```python
from build123d import *

# Parameters (mm, degrees)
F1_DEPTH = 16
F2_T     = -2
F3_W     = 41.64
F3_H     = 10.8
F3_R     = 2.75
F4_DEPTH = 16.001
F5_R     = 1
F6_DEPTH = 5.5


with BuildPart() as f1:
    # F0 (on Top) → F1 (new body)
    with BuildSketch(Plane.XY):
        with BuildLine():
            ThreePointArc((36.115, 24.13), (33.906585, 29.461585), (28.575, 31.67))
            Line((28.575, 31.67), (-28.575, 31.67))
            ThreePointArc((-28.575, 31.67), (-33.906585, 29.461585), (-36.115, 24.13))
            Line((-36.115, 24.13), (-36.115, -24.13))
            ThreePointArc((-36.115, -24.13), (-33.906585, -29.461585), (-28.575, -31.67))
            Line((-28.575, -31.67), (28.575, -31.67))
            ThreePointArc((28.575, -31.67), (33.906585, -29.461585), (36.115, -24.13))
            Line((36.115, -24.13), (36.115, 24.13))
        make_face()
    extrude(amount=F1_DEPTH)

    # F2
    f2_openings = [f1.faces().sort_by_distance(p)[0] for p in [
        (0, 0, 16),
    ]]
    offset(amount=F2_T, openings=f2_openings)

    # F3 (on Top) → F4 (cut, through all)
    with BuildSketch(Plane.XY):
        with Locations((-0.635, -19.162)):
            Rectangle(F3_W, F3_H)
        with BuildLine():
            Line((-8.585, -0.6), (-18.085, -0.6))
            ThreePointArc((-18.085, -0.6), (-18.792107, -0.892893), (-19.085, -1.6))
            Line((-19.085, -1.6), (-19.085, -11.1))
            ThreePointArc((-19.085, -11.1), (-18.792107, -11.807107), (-18.085, -12.1))
            Line((-18.085, -12.1), (-8.585, -12.1))
            ThreePointArc((-8.585, -12.1), (-7.877893, -11.807107), (-7.585, -11.1))
            Line((-7.585, -11.1), (-7.585, -1.6))
            ThreePointArc((-7.585, -1.6), (-7.877893, -0.892893), (-8.585, -0.6))
        make_face()
        with Locations((-26.035, -6.35)):
            Circle(F3_R)
        with BuildLine():
            Line((-8.585, 20.08), (-18.085, 20.08))
            ThreePointArc((-18.085, 20.08), (-18.792107, 19.787107), (-19.085, 19.08))
            Line((-19.085, 19.08), (-19.085, 9.58))
            ThreePointArc((-19.085, 9.58), (-18.792107, 8.872893), (-18.085, 8.58))
            Line((-18.085, 8.58), (-8.585, 8.58))
            ThreePointArc((-8.585, 8.58), (-7.877893, 8.872893), (-7.585, 9.58))
            Line((-7.585, 9.58), (-7.585, 19.08))
            ThreePointArc((-7.585, 19.08), (-7.877893, 19.787107), (-8.585, 20.08))
        make_face()
        with Locations((-26.035, 14.33)):
            Circle(F3_R)
        with BuildLine():
            Line((23.165, -0.6), (13.665, -0.6))
            ThreePointArc((13.665, -0.6), (12.957893, -0.892893), (12.665, -1.6))
            Line((12.665, -1.6), (12.665, -11.1))
            ThreePointArc((12.665, -11.1), (12.957893, -11.807107), (13.665, -12.1))
            Line((13.665, -12.1), (23.165, -12.1))
            ThreePointArc((23.165, -12.1), (23.872107, -11.807107), (24.165, -11.1))
            Line((24.165, -11.1), (24.165, -1.6))
            ThreePointArc((24.165, -1.6), (23.872107, -0.892893), (23.165, -0.6))
        make_face()
        with Locations((5.715, -6.35)):
            Circle(F3_R)
        with BuildLine():
            Line((23.165, 20.08), (13.665, 20.08))
            ThreePointArc((13.665, 20.08), (12.957893, 19.787107), (12.665, 19.08))
            Line((12.665, 19.08), (12.665, 9.58))
            ThreePointArc((12.665, 9.58), (12.957893, 8.872893), (13.665, 8.58))
            Line((13.665, 8.58), (23.165, 8.58))
            ThreePointArc((23.165, 8.58), (23.872107, 8.872893), (24.165, 9.58))
            Line((24.165, 9.58), (24.165, 19.08))
            ThreePointArc((24.165, 19.08), (23.872107, 19.787107), (23.165, 20.08))
        make_face()
        with Locations((5.715, 14.33)):
            Circle(F3_R)
    extrude(amount=F4_DEPTH, mode=Mode.SUBTRACT)

    # F5 (on face) → F6 (join)
    with BuildSketch(Plane.XY.offset(2)):
        with BuildLine():
            Line((-34.115, 24.13), (-34.115, 21.59))
            Line((-34.115, 21.59), (-28.575, 21.59))
            ThreePointArc((-28.575, 21.59), (-26.778949, 22.333949), (-26.035, 24.13))
            Line((-26.035, 24.13), (-26.035, 29.67))
            Line((-26.035, 29.67), (-28.575, 29.67))
            ThreePointArc((-28.575, 29.67), (-32.492372, 28.047372), (-34.115, 24.13))
        make_face()
        with Locations((-28.575, 24.13)):
            Circle(F5_R, mode=Mode.SUBTRACT)
        with BuildLine():
            Line((28.575, 21.59), (34.115, 21.59))
            Line((34.115, 21.59), (34.115, 24.13))
            ThreePointArc((34.115, 24.13), (32.492372, 28.047372), (28.575, 29.67))
            Line((28.575, 29.67), (26.035, 29.67))
            Line((26.035, 29.67), (26.035, 24.13))
            ThreePointArc((26.035, 24.13), (26.778949, 22.333949), (28.575, 21.59))
        make_face()
        with Locations((28.575, 24.13)):
            Circle(F5_R, mode=Mode.SUBTRACT)
        with BuildLine():
            Line((26.035, -24.13), (26.035, -29.67))
            Line((26.035, -29.67), (28.575, -29.67))
            ThreePointArc((28.575, -29.67), (32.492372, -28.047372), (34.115, -24.13))
            Line((34.115, -24.13), (34.115, -21.59))
            Line((34.115, -21.59), (28.575, -21.59))
            ThreePointArc((28.575, -21.59), (26.778949, -22.333949), (26.035, -24.13))
        make_face()
        with Locations((28.575, -24.13)):
            Circle(F5_R, mode=Mode.SUBTRACT)
        with BuildLine():
            Line((-34.115, -21.59), (-34.115, -24.13))
            ThreePointArc((-34.115, -24.13), (-32.492372, -28.047372), (-28.575, -29.67))
            Line((-28.575, -29.67), (-26.035, -29.67))
            Line((-26.035, -29.67), (-26.035, -24.13))
            ThreePointArc((-26.035, -24.13), (-26.778949, -22.333949), (-28.575, -21.59))
            Line((-28.575, -21.59), (-34.115, -21.59))
        make_face()
        with Locations((-28.575, -24.13)):
            Circle(F5_R, mode=Mode.SUBTRACT)
    extrude(amount=F6_DEPTH)


solid = f1.part
```
Check sheet for the modelled part. Datum: model origin and axes. Units: mm. A direction names the side the tool comes from. Give positions to 0.01 mm unless a question says otherwise; leave off trailing zeros. Order: outer loops, then holes, each group sorted by start corner. A loop starts at its lowest first (then second) coordinate and runs counter-clockwise, first axis right, second up. Notation, with made-up numbers: (83, 80.5) -> (120, 80.5) arc R19 ccw to (120, 111.5) -> close; hole circle Ø3 at (50, 47). An arc over 180 degrees is marked (long way). Return JSON: item names as keys, results as strings.
1. Set-up check for faces 4 (the flat face through (-13, 8.58, 1)), 5 (the flat face through (0, 31, 16)), 6 (the flat face through (-31, -21.59, 5)): record each of +Z, -Z, +X, -X, +Y, -Y from which the full face is reachable in a straight line by a thin tool's end or side.
From the geometry:
{"face 4": "+Z, -Z", "face 5": "+Z, +X, -X, +Y, -Y", "face 6": "+Z"}
2. Material ranges on probe 1 along X at (y, z) = (-6.35, 0.6) (3 decimals); probe 2 along Y at (x, z) = (8.5, 14.25); probe 3 along X at (y, z) = (-9, 7.75) (3 decimals), recorded low to high. Write a range as [from, to].
From the geometry:
{"probe 1": "[-36.115, -28.785], [-23.285, -19.085], [-7.585, 2.965], [8.465, 12.665], [24.165, 36.115]", "probe 2": "[-31.67, -29.67], [29.67, 31.67]", "probe 3": "[-36.115, -34.115], [34.115, 36.115]"}
3. Go/stop test with flat-tipped pins: P1, Ø5, axis at x = 15.5, y = -19.5, coming from the +Z side; P2, Ø2, axis at x = -29, y = -24, coming from the +Z side; P3, Ø6, axis at x = -26, y = -12.5, coming from the +Z side. Record where each tip stops, or that it passes through.
From the geometry:
{"P1": "through", "P2": "z = 7.5", "P3": "z = 2"}
4. Cross-section at B-B, the plane x = -15. Record the cut outline in (y, z).
From the geometry:
{"outline": "(-31.67, 0) -> (-24.56, 0) -> (-24.56, 2) -> (-29.67, 2) -> (-29.67, 16) -> (-31.67, 16) -> close; (-13.76, 0) -> (-12.1, 0) -> (-12.1, 2) -> (-13.76, 2) -> close; (-0.6, 0) -> (8.58, 0) -> (8.58, 2) -> (-0.6, 2) -> close; (20.08, 0) -> (31.67, 0) -> (31.67, 16) -> (29.67, 16) -> (29.67, 2) -> (20.08, 2) -> close"}
5. Mould release check, pull along Y, two halves, no side actions. Record for faces 1 (the flat face through (12.665, -6, 1)), 2 (the cylindrical face through (-33.85, 29.52, 7.89)), 3 (the flat face through (36.115, 0, 8)): +Y half, -Y half, draft (parallel to the pull), parting line (faces both ways), or undercut.
From the geometry:
{"face 1": "undercut", "face 2": "+Y half", "face 3": "draft"}
6. Cross-section at A-A, the plane z = 12. Record the cut outline in (x, y) (3 decimals).
From the geometry:
{"outline": "(-36.115, -24.13) arc R7.54 ccw to (-28.575, -31.67) -> (28.575, -31.67) arc R7.54 ccw to (36.115, -24.13) -> (36.115, 24.13) arc R7.54 ccw to (28.575, 31.67) -> (-28.575, 31.67) arc R7.54 ccw to (-36.115, 24.13) -> close; hole (-34.115, -24.13) arc R5.54 ccw to (-28.575, -29.67) -> (28.575, -29.67) arc R5.54 ccw to (34.115, -24.13) -> (34.115, 24.13) arc R5.54 ccw to (28.575, 29.67) -> (-28.575, 29.67) arc R5.54 ccw to (-34.115, 24.13) -> close"}
7. Cross-section at D-D, the plane z = 4. Record the cut outline in (x, y) (3 decimals).
From the geometry:
{"outline": "(-36.115, -24.13) arc R7.54 ccw to (-28.575, -31.67) -> (28.575, -31.67) arc R7.54 ccw to (36.115, -24.13) -> (36.115, 24.13) arc R7.54 ccw to (28.575, 31.67) -> (-28.575, 31.67) arc R7.54 ccw to (-36.115, 24.13) -> close; hole (-34.115, -21.59) -> (-28.575, -21.59) arc R2.54 cw to (-26.035, -24.13) -> (-26.035, -29.67) -> (26.035, -29.67) -> (26.035, -24.13) arc R2.54 cw to (28.575, -21.59) -> (34.115, -21.59) -> (34.115, 21.59) -> (28.575, 21.59) arc R2.54 cw to (26.035, 24.13) -> (26.035, 29.67) -> (-26.035, 29.67) -> (-26.035, 24.13) arc R2.54 cw to (-28.575, 21.59) -> (-34.115, 21.59) -> close; hole circle Ø2 at (-28.575, -24.13); hole circle Ø2 at (-28.575, 24.13); hole circle Ø2 at (28.575, -24.13); hole circle Ø2 at (28.575, 24.13)"}
8. Cross-section at C-C, the plane y = -16. Record the cut outline in (x, z) (3 decimals).
From the geometry:
{"outline": "(-36.115, 0) -> (-21.455, 0) -> (-21.455, 2) -> (-34.115, 2) -> (-34.115, 16) -> (-36.115, 16) -> close; (20.185, 0) -> (36.115, 0) -> (36.115, 16) -> (34.115, 16) -> (34.115, 2) -> (20.185, 2) -> close"}
